The model under review builds one solid part; all positions refer to its coordinate system, in mm. A direction names the side the tool comes from. Coordinates: 2 decimals unless noted, no trailing zeros. Order: outer loops, then holes, each group sorted by start corner. A loop starts at its lowest first (then second) coordinate and runs counter-clockwise, first axis right, second up. Notation, with made-up numbers: (89, 11.5) -> (105, 11.5) arc R14 ccw to (105, 24.5) -> close; hole circle Ø8 at (43.25, -12.75). An arc over 180 degrees is marked (long way). Put each result on its own line as item: value.
from build123d import *

# Parameters (mm, degrees)
F1_DEPTH = 63.5
F0_W     = 25.2737943477
F0_H     = 19.05
F2_DEPTH = 25.4
F3_DEPTH = 7.9375


with BuildPart() as f1:
    # F0 (on Front) → F1 (new body, symmetric)
    with BuildSketch(Plane.XZ):
        Polygon((-41.275, 9.525), (-41.275, -9.525), (41.275, -9.525), (41.275, 9.525), (22.225, 9.525), align=None)
    extrude(amount=F1_DEPTH, both=True)

    # F0 (on Front) → F2 (join, symmetric)
    with BuildSketch(Plane.XZ):
        with BuildLine():
            Line((22.225, 9.525), (41.275, 9.525))
            Line((41.275, 9.525), (41.275, 27.0002))
            ThreePointArc((41.275, 27.0002), (45.9246798487, 38.2255201513), (57.15, 42.8752))
            Line((57.15, 42.8752), (60.325, 42.8752))
            Line((60.325, 42.8752), (60.325, 61.9252))
            Line((60.325, 61.9252), (57.15, 61.9252))
            ThreePointArc((57.15, 61.9252), (32.4542956671, 51.6959043329), (22.225, 27.0002))
            Line((22.225, 27.0002), (22.225, 9.525))
        make_face()
        with Locations((72.9618971738, 52.4002)):
            Rectangle(F0_W, F0_H)
    extrude(amount=F2_DEPTH, both=True)

    # F0 (on Front) → F3 (join, symmetric)
    with BuildSketch(Plane.XZ):
        with BuildLine():
            add(Edge.make_bspline(
                [(-41.275, 9.525), (-41.1781184375, 34.5562882721), (9.094000794, 62.791056931), (57.15, 61.9252)],
                knots=[0, 0, 0, 0, 111.5045361635, 111.5045361635, 111.5045361635, 111.5045361635], degree=3))
            Line((-41.275, 9.525), (22.225, 9.525))
            Line((22.225, 9.525), (22.225, 27.0002))
            ThreePointArc((22.225, 27.0002), (32.4542956671, 51.6959043329), (57.15, 61.9252))
        make_face()
    extrude(amount=F3_DEPTH, both=True)

    # F0 (on Front) → F4 (revolve)
    with BuildSketch(Plane.XZ):
        Polygon((85.5987943477, 66.675), (85.5987943477, 61.9252), (85.5987943477, 42.8752), (85.5987943477, 38.1), (111.125, 38.1), (111.125, 66.675), align=None)
    revolve(axis=Axis((85.5987943477, 0, 52.3875), (0, 0, 1)))


solid = f1.part
Item 1: Mouldability with a two-part tool opening along X and no side actions: class faces 1 (the flat face through (41.275, -1, 4)), 2 (the flat face through (-1, -63.5, 0)), 3 (the flat face through (59, 4, 42.875)), 4 (the cylindrical face through (32.73, -16.79, 51.97)) as +X half, -X half, draft (parallel to the pull), parting line (faces both ways), or undercut.
Answers below:
face 1: +X half
face 2: draft
face 3: undercut
face 4: -X half
Item 2: Consider section A-A on z = 6. Write out the cut boundary in (x, y) (3 decimals), and give its area (3 significant figures).
Answers below:
outline: (-41.275, -63.5) -> (41.275, -63.5) -> (41.275, 63.5) -> (-41.275, 63.5) -> close
area: 10,500 mm^2
Item 3: For line 1 (X direction, y = 3, z = 9) (3 decimals); line 2 (X direction, y = 18, z = 24) (3 decimals); line 3 (Z direction, x = 3, y = 58) (3 decimals), list the stretches that pass through material, from the lowest coordinate up. Write a range as from..to.
Answers below:
line 1: -41.275..41.275
line 2: 22.225..41.275
line 3: -9.525..9.525
Item 4: Consider section B-B on y = 12. Write out the cut boundary in (x, z) (3 decimals).
Answers below:
outline: (-41.275, -9.525) -> (41.275, -9.525) -> (41.275, 27) arc R15.875 cw to (57.15, 42.875) -> (63.069, 42.875) -> (63.069, 38.1) -> (108.128, 38.1) -> (108.128, 66.675) -> (63.069, 66.675) -> (63.069, 61.925) -> (57.15, 61.925) arc R34.925 ccw to (22.225, 27) -> (22.225, 9.525) -> (-41.275, 9.525) -> close
Item 5: Consider section C-C on x = 98.5. Write out the cut boundary in (y, z) (3 decimals).
Answers below:
outline: (-22.026, 38.1) -> (22.026, 38.1) -> (22.026, 66.675) -> (-22.026, 66.675) -> close
Item 6: For faces 5 (the flat face through (22.225, -17, 18)), 6 (the cylindrical face through (32.73, 16.55, 51.97)), 7 (the flat face through (60, 2, 61.925)), 8 (the flat face through (86, 0, 38.1)), list the 3-axis set-ups (+Z, -Z, +X, -X, +Y, -Y) from which the entire face can be reached by the end or side of a thin tool; tool diameter is ignored.
Answers below:
face 5: +Z, -X, -Y
face 6: +Z, -X, +Y
face 7: +Z, -X
face 8: -Z, +X, +Y, -Y
Item 7: For pin 1 Ø3 at (x, y) = (56, -26.5) entering from -Z; pin 2 Ø4 at (x, z) = (4, 10.5) entering from +Y; pin 3 Ø1.5 at (x, y) = (1, -22) entering from +Z (3 decimals); pin 4 Ø8 at (x, y) = (68, 3) entering from -Z, all flat-tipped, find the tip position at first contact; note any pin that passes through.
Answers below:
pin 1: z = 42.73
pin 2: y = 63.5
pin 3: z = 9.525
pin 4: z = 38.1
